The listing builds one solid part. Answer for the finished solid, in the listing's coordinates (mm). A direction names the side the tool comes from. Coordinates: 2 decimals unless noted, no trailing zeros. Write each loop counter-clockwise with the first axis right and the second up, starting at its lowest first coordinate (ties: lowest second). Pieces come first, ordered by that corner, then holes.
(1) Given P1, Ø16.5, axis at y = 0, z = 0, coming from the -X side; P2, Ø5, axis at x = 22, y = -14, coming from the +Z side; P3, Ø12, axis at x = 18, y = -16.5, coming from the -Z side; P4, Ø3, axis at x = 36, y = 2, coming from the +Z side, each flat-ended and moving along its own axis, determine where each tip first touches the part or whether it passes through.
(2) Straight lines are drawn through the part: line 1 (Y direction, x = 38, z = 0); line 2 (Z direction, x = 39, y = 0). For each, find the intervals that lie inside material, in ascending order.
(3) Which of the six approach directions +Z, -Z, +X, -X, +Y, -Y give full straight-line access (tool end or side, diameter ignored) to faces 4 (the conical face through (47.165, -1.855, 16.162)), 5 (the flat face through (19.05, -9.4, 9.4)), 6 (the cylindrical face through (53.131, -4.627, 20.835))?
(4) For a pull along X with two mould halves and no side action, classify faces 1 (the cylindrical face through (14.699, -2.449, 11.028)), 2 (the cylindrical face through (30.96, 1.926, -6.117)), 3 (the flat face through (60.325, 5, -5)) as +X half, -X half, draft (parallel to the pull), parting line (faces both ways), or undercut.
(5) The part is cut by section A-A on x = 56. Determine the outline of the cut face in (y, z), plus the area to 3 significant figures.
(6) The part is cut by section B-B on y = 0. Give the number of separate pieces and of enclosed holes in the cut face, plus the area to 3 significant figures.
from build123d import *

# Parameters (mm, degrees)
HOLE1_D           = 12.827
HOLE1_DEPTH       = 60.325
HOLE1_CSINK_D     = 14.351
HOLE1_CSINK_ANGLE = 90


with BuildPart() as part:
    # Sketch1 → Revolve1 (revolve)
    with BuildSketch(Plane.XY):
        with BuildLine():
            Line((0, 0), (0, 11.43127))
            Line((0, 11.43127), (1.26873, 12.7))
            Line((1.26873, 12.7), (11.786186437, 12.7))
            Line((11.786186437, 12.7), (13.129150664, 11.570773334))
            ThreePointArc((13.129150664, 11.570773334), (13.480921475, 11.367317925), (13.8811, 11.29665))
            Line((13.8811, 11.29665), (15.494, 11.29665))
            ThreePointArc((15.494, 11.29665), (16.320183563, 11.638866437), (16.6624, 12.46505))
            Line((16.6624, 12.46505), (16.6624, 13.08735))
            Line((16.6624, 13.08735), (19.05, 13.08735))
            Line((19.05, 13.08735), (19.05, 0))
            Line((19.05, 0), (0, 0))
        make_face()
    revolve(axis=Axis((19.05, 0, 0), (-1, 0, 0)))

    # Sketch2 → Revolve2 (revolve)
    with BuildSketch(Plane.XY):
        Polygon((19.05, 0), (19.05, 21.90115), (20.574, 23.42515), (52.3367, 23.42515), (52.3367, 21.34235), (53.3908, 21.34235), (54.4449, 22.39645), (59.563, 22.39645), (60.325, 21.63445), (60.325, 0), align=None)
    revolve(axis=Axis((60.325, 0, 0), (-1, 0, 0)))

    # Hole1
    with Locations(Plane.ZY):
        with Locations((0, 0)):
            CounterSinkHole(HOLE1_D / 2, HOLE1_CSINK_D / 2, depth=HOLE1_DEPTH, counter_sink_angle=HOLE1_CSINK_ANGLE)

    # Sketch5 → Cut-Revolve1 (revolve, cut)
    with BuildSketch(Plane(origin=(0, 0, 0), x_dir=(1, 0, 0), z_dir=(0, 1, 0))):
        Polygon((41.275, 0), (44.45, 0), (44.45, -5.926053545), (47.217096455, -8.69315), (47.677022746, -23.42515), (41.275, -23.42515), align=None)
    revolve(axis=Axis((41.275, 0, 23.42515), (0, 0, -1)), mode=Mode.SUBTRACT)

    # Sketch6 → Revolve3 (revolve)
    with BuildSketch(Plane.XY):
        with BuildLine():
            Line((52.3367, 21.08835), (53.3908, 21.08835))
            Line((53.3908, 21.08835), (53.3908, 21.34235))
            Line((53.3908, 21.34235), (52.86375, 21.34235))
            Line((52.86375, 21.34235), (52.471716303, 21.734383697))
            ThreePointArc((52.471716303, 21.734383697), (52.434518864, 21.824186258), (52.471716303, 21.913988819))
            Line((52.471716303, 21.913988819), (53.898709288, 23.340981804))
            Line((53.898709288, 23.340981804), (53.898709288, 23.42515))
            Line((53.898709288, 23.42515), (53.695509288, 23.42515))
            Line((53.695509288, 23.42515), (52.3367, 22.066340712))
            Line((52.3367, 22.066340712), (52.3367, 21.08835))
        make_face()
    revolve(axis=Axis((53.3908, 0, 0), (-1, 0, 0)))


solid = part.part
Model answer:
1. P1: stops at x = 0
1. P2: stops at z = 20.41
1. P3: stops at z = -20.64
1. P4: stops at z = 23.41
2. line 1: y = -23.43 to -6.41, 6.41 to 23.43
2. line 2: z = -23.43 to -6.41
3. face 4: +Z
3. face 5: -X
3. face 6: none
4. face 1: undercut
4. face 2: draft
4. face 3: +X half
5. outline: circle Ø44.79 at (0, 0); hole circle Ø12.83 at (0, 0)
5. area: 1,450 mm2
6. separate pieces: 3
6. enclosed holes: 0
6. area: 1,410 mm2
